```python
from build123d import *

# Parameters (mm, degrees)
BOSS_EXTRUDE1_DEPTH      = 40.5
BOSS_EXTRUDE1_DEPTH_BACK = 4.5
CUT_EXTRUDE2_DEPTH       = 42.117666519


with BuildPart() as part:
    # Sketch1 → Boss-Extrude1 (new, two sides: drawn at the far end of the back side and taken through both)
    with BuildSketch(Plane(origin=(0, 0, 0), x_dir=(0, 0, -1), z_dir=(1, 0, 0)).offset(-BOSS_EXTRUDE1_DEPTH_BACK)):
        with BuildLine():
            Line((-2.626785107, 2.95), (2.626785107, 2.95))
            ThreePointArc((2.626785107, 2.95), (3.95, 0), (2.626785107, -2.95))
            Line((2.626785107, -2.95), (-2.626785107, -2.95))
            ThreePointArc((-2.626785107, -2.95), (-3.95, 0), (-2.626785107, 2.95))
        make_face()
    extrude(amount=BOSS_EXTRUDE1_DEPTH + BOSS_EXTRUDE1_DEPTH_BACK)

    # Sketch5 → Cut-Extrude2 (cut, through all)
    with BuildSketch(Plane(origin=(0, 2.95, 0), x_dir=(1, 0, 0), z_dir=(0, 1, 0))):
        Polygon((40.5, 0), (40.5, 1), (20, 1), (20, -1), (40.5, -1), align=None)
    extrude(amount=-CUT_EXTRUDE2_DEPTH, mode=Mode.SUBTRACT)


solid = part.part
```
Source: CAD feature listing. Evaluate the final solid. Frame: model axes, mm. A direction names the side the tool comes from. Give positions to 0.01 mm unless a question says otherwise; leave off trailing zeros. Loops run counter-clockwise (first coordinate to the right, second up) from the corner with the lowest first, then second, coordinate; pieces in that order, holes last. Notation, with made-up numbers: (80.25, 33.5) - (120.25, 33.5) arc R11 cw to (120.25, 39.5) - close; hole circle Ø9 at (33.25, -4). An arc over 180 degrees is marked (long way). Use CSV: the item, a comma, the result in double quotes.
1) Line query: line 1 (Z direction, x = 34, y = 1.05); line 2 (X direction, y = 2.65, z = 0.75); line 3 (Z direction, x = 28, y = -0.7). Output: solid intervals per line, ascending.
Worked out:
line 1,"z = -3.81 to -1, 1 to 3.81"
line 2,"x = -4.5 to 20"
line 3,"z = -3.89 to -1, 1 to 3.89"
2) Cut plane C-C (x = 16.5). Output: boundary loops of the cut face in (y, z).
Worked out:
outline,"(-2.95, -2.63) arc R3.95 ccw to (2.95, -2.63) - (2.95, 2.63) arc R3.95 ccw to (-2.95, 2.63) - close"
3) Cut plane A-A (x = 36). Output: boundary loops of the cut face in (y, z).
Worked out:
outline,"(-2.95, -2.63) arc R3.95 ccw to (2.95, -2.63) - (2.95, -1) - (-2.95, -1) - close; (-2.95, 1) - (2.95, 1) - (2.95, 2.63) arc R3.95 ccw to (-2.95, 2.63) - close"
4) Cut plane B-B (y = -2). Output: boundary loops of the cut face in (x, z).
Worked out:
outline,"(-4.5, -3.41) - (40.5, -3.41) - (40.5, -1) - (20, -1) - (20, 1) - (40.5, 1) - (40.5, 3.41) - (-4.5, 3.41) - close"
5) Set-up query: faces 1 (the flat face through (40.5, 0, -2)), 2 (the flat face through (20, 0, 0)). Return all of +Z, -Z, +X, -X, +Y, -Y with unobstructed straight access to the full face (end or side cutting, diameter ignored); none if empty.
Worked out:
face 1,"+Z, -Z, +X, +Y, -Y"
face 2,"+X, +Y, -Y"
6) Pin query (flat end, axial travel): P1, Ø1, axis at x = 3.5, y = 2, coming from the +Z side; P2, Ø1, axis at y = -2, z = 0, coming from the +X side. Return the tip coordinate at first contact, or that it passes through.
Worked out:
P1,"stops at z = 3.65"
P2,"stops at x = 20"
7) Cut plane D-D (z = 0.5). Output: boundary loops of the cut face in (x, y).
Worked out:
outline,"(-4.5, -2.95) - (20, -2.95) - (20, 2.95) - (-4.5, 2.95) - close"
8) Mould query, pull axis Z, two halves, no side actions, for faces 3 (the flat face through (18, 2.95, 0)), 4 (the flat face through (30, 0, -1)), 5 (the cylindrical face through (17.68, -0.05, 3.95)). Classes: +Z half, -Z half, draft (parallel to the pull), parting line (faces both ways), or undercut.
Worked out:
face 3,"draft"
face 4,"undercut"
face 5,"+Z half"
